For this review, take the finished solid that the model builds, in its own axes (mm). A direction names the side the tool comes from. Give positions to 0.01 mm unless a question says otherwise; leave off trailing zeros. Write each loop counter-clockwise with the first axis right and the second up, starting at its lowest first coordinate (ties: lowest second). Pieces come first, ordered by that corner, then holes. Notation, with made-up numbers: M 0,-33 L 21,-33 A18 cw 21,-3 Z; hole C 43.25,62.5 d10. An arc over 180 degrees is marked long. Write item = value, one per line.
```python
from build123d import *

# Parameters (mm, degrees)
EXTRUDE_1_DEPTH        = 356
HOLE_WIZARD_M5_1_D     = 4.2
HOLE_WIZARD_M5_1_DEPTH = 12
HOLE_WIZARD_M5_1_TIP   = 1.2618073
SKETCH_13_R            = 4.5
CUT_EXTRUDE_1_DEPTH    = 384.170980112
HOLE_WIZARD_M4_1_D     = 3.3
PATTERN_LINEAR_1_COUNT = 6
PATTERN_LINEAR_1_PITCH = 60
HOLE_WIZARD_M5_2_D     = 4.2
HOLE_WIZARD_M5_2_DEPTH = 12
HOLE_WIZARD_M5_2_TIP   = 1.2618073


with BuildPart() as part:
    # 草图1 → 凸台-拉伸1 (new body)
    with BuildSketch(Plane(origin=(0, 0, 0), x_dir=(0, 0, -1), z_dir=(1, 0, 0))):
        Polygon((0, 0), (32, 0), (32, -20), (10, -20), (10, -120), (32, -120), (32, -140), (0, -140), align=None)
    extrude(amount=EXTRUDE_1_DEPTH)

    # M5 螺纹孔1
    with Locations(Plane(origin=(356, -130, -25), x_dir=(0, 0, 1), z_dir=(1, 0, 0))):
        with Locations((0, 0), (18, 0), (18, -120), (0, -120), (20, -60)):
            Hole(HOLE_WIZARD_M5_1_D / 2, depth=HOLE_WIZARD_M5_1_DEPTH)
            with Locations((0, 0, -(HOLE_WIZARD_M5_1_DEPTH + HOLE_WIZARD_M5_1_TIP / 2))):  # 118° drill point
                Cone(0, HOLE_WIZARD_M5_1_D / 2, HOLE_WIZARD_M5_1_TIP, mode=Mode.SUBTRACT)

    # 草图13 → 切除-拉伸1 (cut, through all)
    with BuildSketch(Plane(origin=(0, 0, -10), x_dir=(-1, 0, 0), z_dir=(0, 0, -1))):
        with Locations(Location((-346, -44, 0), (0, 0, 90))):
            Circle(SKETCH_13_R)
        with Locations(Location((-346, -96, 0), (0, 0, 90))):
            Circle(SKETCH_13_R)
        with Locations(Location((-54.5, -44, 0), (0, 0, 90))):
            Circle(SKETCH_13_R)
        with Locations(Location((-54.5, -96, 0), (0, 0, 90))):
            Circle(SKETCH_13_R)
    extrude(amount=-CUT_EXTRUDE_1_DEPTH, mode=Mode.SUBTRACT)

    # M4 螺纹孔1 (through all)
    with Locations(Plane(origin=(328, -130, -32), x_dir=(-1, 0, 0), z_dir=(0, 0, -1))):
        with Locations((0, 0), (0, 120)):
            hole_wizard_m4_1 = Hole(HOLE_WIZARD_M4_1_D / 2)

    # 阵列(线性)1: M4 螺纹孔1 ×6
    with Locations(*[(-i * PATTERN_LINEAR_1_PITCH, 0, 0) for i in range(1, PATTERN_LINEAR_1_COUNT)]):
        add(hole_wizard_m4_1, mode=Mode.SUBTRACT)

    # M5 螺纹孔2
    with Locations(Plane.ZY):
        with Locations((-7, -10), (-25, -10), (-5, -70), (-7, -130), (-25, -130)):
            Hole(HOLE_WIZARD_M5_2_D / 2, depth=HOLE_WIZARD_M5_2_DEPTH)
            with Locations((0, 0, -(HOLE_WIZARD_M5_2_DEPTH + HOLE_WIZARD_M5_2_TIP / 2))):  # 118° drill point
                Cone(0, HOLE_WIZARD_M5_2_D / 2, HOLE_WIZARD_M5_2_TIP, mode=Mode.SUBTRACT)


solid = part.part
```
1. We need section B-B, the plane y = -44. Write out the cut boundary in (x, z).
Responses:
outline = M 0,-10 L 50,-10 L 50,0 L 0,0 Z; M 59,-10 L 341.5,-10 L 341.5,0 L 59,0 Z; M 350.5,-10 L 356,-10 L 356,0 L 350.5,0 Z
2. We need section D-D, the plane y = -87. Write out the cut boundary in (x, z).
Responses:
outline = M 0,-10 L 356,-10 L 356,0 L 0,0 Z
3. We need section A-A, the plane z = -15. Count the separate pieces of the cut face and the enclosed holes in it, then the cut area to 3 significant figures.
Responses:
separate_pieces = 2
enclosed_holes = 12
area = 14,100 mm2
4. The part is to be moulded in two halves that separate along X. For faces 3 (the face through (0, -69, -9)), 4 (the face through (176, -120, -21)), 5 (the face through (342.01, -41.92, -5.07)), 6 (the face through (50.51, -41.92, -5.07)), say which applies: +X half, -X half, draft (parallel to the pull), parting line (faces both ways), or undercut.
Responses:
face_3 = -X half
face_4 = draft
face_5 = undercut
face_6 = undercut
5. Insertion check: P1, Ø2.5, axis at x = 328, y = -10, coming from the +Z side; P2, Ø12, axis at x = 233, y = -61.5, coming from the -Z side; P3, Ø2.5, axis at y = -130, z = -25, coming from the -X side; P4, Ø2.5, axis at y = -10, z = -7, coming from the +X side. Each pin has a flat end and moves straight along its axis. Give the tip position at first contact, or say it passes through.
Responses:
P1 = through
P2 = -10
P3 = 12.51
P4 = 343.49
6. For line 1 along Y through (x, z) = (88, -23); line 2 along Z through (x, y) = (8.5, -10); line 3 along Z through (x, y) = (7, -70), list the stretches that pass through material, from the lowest coordinate up. Write a range as from..to.
Responses:
line_1 = -140..-131.65, -128.35..-120, -20..-11.65, -8.35..0
line_2 = -32..-27.1, -22.9..-9.1, -4.9..0
line_3 = -10..-7.1, -2.9..0
7. We need section C-C, the plane x = 94.5. Write out the cut boundary in (y, z).
Responses:
outline = M -140,-32 L -120,-32 L -120,-10 L -20,-10 L -20,-32 L 0,-32 L 0,0 L -140,0 Z
8. Machinability: for faces 1 (the face through (51.8, -99.6, -5.1)), 2 (the face through (176, -69, -10)), which of the approach directions +Z, -Z, +X, -X, +Y, -Y give a long, thin tool a straight path to every point of the face, cutting with its end or side? Answer none if there is none.
Responses:
face_1 = +Z, -Z
face_2 = -Z, +X, -X
